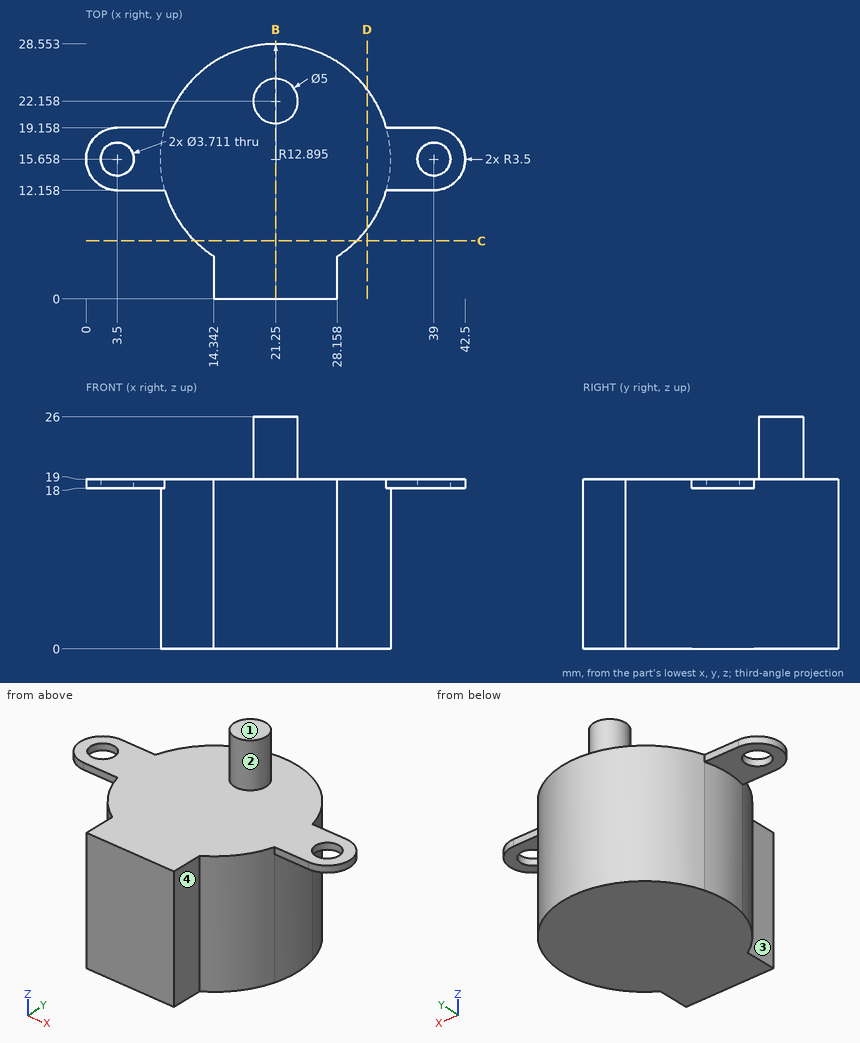
Geometry: see drawing. Coordinates: mm, zero at the bounding-box minimum. A direction names the side the tool comes from. Coordinates: 2 decimals unless noted, no trailing zeros. Order: outer loops, then holes, each group sorted by start corner. A loop starts at its lowest first (then second) coordinate and runs counter-clockwise, first axis right, second up. Notation, with made-up numbers: M -34.75,38.5 L -20.75,38.5 A26 cw -20.75,70.5 Z; hole C -20.75,75.25 d1. An arc over 180 degrees is marked long. Answer in a Markdown table with one row per item. Add a question column.
Q1. Reachability of the marked faces 1, 2, 3 and 4 from +Z, -Z, +X, -X, +Y, -Y: full face, straight path, thin tool, end or side. Return the list, or none.
Q2. Section query C-C on y = 6.5. Return the cut outline in (x, z), and give its area (3 significant figures).
Q3. Section query B-B on x = 21.25. Return the cut outline in (y, z).
Q4. Contact query for flat-ended pins moving along their axis: P1, Ø0.8, axis at x = 37, z = 18.5, coming from the -Y side; P2, Ø4, axis at y = 2, z = 12, coming from the -X side; P3, Ø2, axis at x = 6, y = 14.5, coming from the -Z side; P4, Ø1.5, axis at x = 17, z = 22, coming from the -Y side. Output: stop coordinate, or through.
Q5. Section query D-D on x = 31.5. Return the cut outline in (y, z) (1 decimal).
Q6. Line query: L1, parallel to Y at x = 39, z = 18.6; L2, parallel to Z at x = 17.5, y = 7; L3, parallel to X at y = 2.5, z = 15.25. Output: solid intervals per line, ascending.
Completed:
| question | item | result |
|---|---|---|
| 1 | face 1 | +Z, +X, -X, +Y, -Y |
| 1 | face 2 | +Z |
| 1 | face 3 | +Z, -Z, -X, -Y |
| 1 | face 4 | +Z, -Z, +X, -Y |
| 2 | outline | M 12.17,0 L 30.33,0 L 30.33,19 L 12.17,19 Z |
| 2 | area | 345 mm2 |
| 3 | outline | M 0,0 L 28.55,0 L 28.55,19 L 24.66,19 L 24.66,26 L 19.66,26 L 19.66,19 L 0,19 Z |
| 4 | P1 | stops at y = 12.16 |
| 4 | P2 | stops at x = 14.34 |
| 4 | P3 | stops at z = 18 |
| 4 | P4 | passes through |
| 5 | outline | M 7.8,0 L 23.5,0 L 23.5,19 L 7.8,19 Z |
| 6 | L1 | y = 12.16 to 13.8, 17.51 to 19.16 |
| 6 | L2 | z = 0 to 19 |
| 6 | L3 | x = 14.34 to 28.16 |
